Here's how the part is built. I have some questions about the finished solid (model axes, mm). Face numbers are marked on the shaded views. A direction names the side the tool comes from. Give positions to 0.01 mm unless a question says otherwise; leave off trailing zeros. Loops run counter-clockwise (first coordinate to the right, second up) from the corner with the lowest first, then second, coordinate; pieces in that order, holes last. Notation, with made-up numbers: (27, 82) - (52, 82) arc R12 cw to (52, 100) - close; hole circle Ø2 at (25.25, 39.25). An arc over 180 degrees is marked (long way). Return JSON: item names as keys, results as strings. Group by question number.
(1) If we section it at C-C (y = -10): Please give me the cut outline in (x, z), then the cut area to 3 significant figures.
(2) On a 3-axis mill with a long thin cutter (end or side, diameter ignored), from which of +Z, -Z, +X, -X, +Y, -Y can I reach the whole of each face in a straight line? I mean the marked faces 4 and 5. Say none if no direction works.
(3) If we mould it in two halves opening along X, with no side actions, what happens to the marked faces 1, 2 and 3? For each: released by +X, released by -X, zero draft, split by the parting line, or undercut.
(4) For P1, Ø12, axis at y = 147, z = -54.5, coming from the -X side; P2, Ø5, axis at x = 144.5, z = -67, coming from the -Y side; P3, Ø3, axis at x = 94.5, z = -38, coming from the +Y side; P4, Ø2, axis at x = -243.5, y = 81, coming from the +Z side, each with a flat end and sliding along its axis, tell me the tip position at first contact or that it passes through.
(5) I need wall thicknesses on probe 1 along Y at (x, z) = (0, -30.5); probe 2 along Y at (x, z) = (23.5, -88.5); probe 3 along X at (y, z) = (0, -37). Which ranges of each line are inside material? Lowest first, please. Write a range as [from, to].
(6) If we section it at A-A (x = 0): Please give me the cut outline in (y, z), then the cut area to 3 significant figures.
(7) If we section it at B-B (z = -100): Please give me the cut outline in (x, y), then the cut area to 3 significant figures.
(8) If we section it at D-D (x = -199): Please give me the cut outline in (y, z).
```python
from build123d import *

# Parameters (mm, degrees)
F1_DEPTH = 150
F3_DEPTH = 264.16


with BuildPart() as f1:
    # F0 (on Top) → F1 (new body)
    with BuildSketch(Plane.XY):
        with BuildLine():
            ThreePointArc((-261.9368960265, 146.25), (-75.5610057902, -290.3283217393), (300, 0))
            ThreePointArc((300, 0), (290.3283217393, 75.5610057902), (261.9368960265, 146.25))
            ThreePointArc((261.9368960265, 146.25), (0, 295), (-261.9368960265, 146.25))
        make_face()
        with BuildLine():
            ThreePointArc((261.9368960265, 146.25), (290.3283217393, 75.5610057902), (300, 0))
            ThreePointArc((300, 0), (-75.5610057902, -290.3283217393), (-261.9368960265, 146.25))
            ThreePointArc((-261.9368960265, 146.25), (-81.0377896784, -304.0372028231), (305, -10))
            ThreePointArc((305, -10), (294.0372028231, 71.0377896784), (261.9368960265, 146.25))
        make_face()
        with BuildLine():
            ThreePointArc((-261.9368960265, 146.25), (0, 295), (261.9368960265, 146.25))
            ThreePointArc((261.9368960265, 146.25), (0, 300), (-261.9368960265, 146.25))
        make_face()
    extrude(amount=-F1_DEPTH)

    # F2 (on Top) → F3 (cut)
    with BuildSketch(Plane.XY):
        with BuildLine():
            ThreePointArc((-40, 118.4271928233), (-72.8868986856, -101.5504800579), (125, 0))
            ThreePointArc((125, 0), (101.5504800579, 72.8868986856), (40, 118.4271928233))
            Line((40, 118.4271928233), (40, 0))
            Line((40, 0), (-40, 0))
            Line((-40, 0), (-40, 118.4271928233))
        make_face()
        with BuildLine():
            Line((40, 0), (40, 118.4271928233))
            ThreePointArc((40, 118.4271928233), (0, 125), (-40, 118.4271928233))
            Line((-40, 118.4271928233), (-40, 0))
            Line((-40, 0), (40, 0))
        make_face()
        with BuildLine():
            ThreePointArc((-40, 118.4271928233), (0, 125), (40, 118.4271928233))
            Line((40, 118.4271928233), (40, 158))
            Line((40, 158), (-40, 158))
            Line((-40, 158), (-40, 118.4271928233))
        make_face()
    extrude(amount=-F3_DEPTH, mode=Mode.SUBTRACT)


solid = f1.part
```
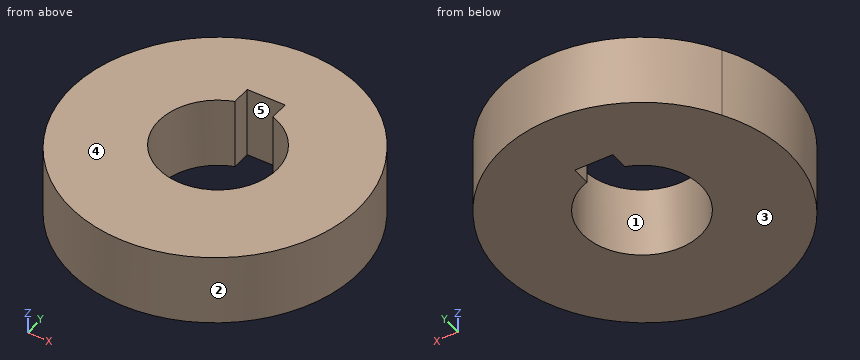
Values:
{
 "1": {"outline": "(-305, -150) - (-124.6, -150) - (-124.6, 0) - (-305, 0) - close; (124.6, -150) - (305, -150) - (305, 0) - (124.6, 0) - close", "area": "54,100 mm2"},
 "2": {"face 4": "+Z, +X, -X, +Y, -Y", "face 5": "+Z, -Z"},
 "3": {"face 1": "undercut", "face 2": "split by the parting line", "face 3": "zero draft"},
 "4": {"P1": "x = -265", "P2": "y = -279.93", "P3": "y = 285.22", "P4": "z = 0"},
 "5": {"probe 1": "[-315, -125], [158, 300]", "probe 2": "[-314.09, -122.77], [158, 299.08]", "probe 3": "[-304.84, -125], [125, 304.84]"},
 "6": {"outline": "(-315, -150) - (-125, -150) - (-125, 0) - (-315, 0) - close; (158, -150) - (300, -150) - (300, 0) - (158, 0) - close", "area": "49,800 mm2"},
 "7": {"outline": "(-261.94, 146.25) arc R305 ccw (long way) to (261.94, 146.25) arc R300 ccw to start; hole (-40, 118.43) arc R125 ccw (long way) to (40, 118.43) - (40, 158) - (-40, 158) - close", "area": "242,000 mm2"},
 "8": {"outline": "(-241.14, -150) - (224.5, -150) - (224.5, 0) - (-241.14, 0) - close"}
}
